Part model, mm, in its own coordinate system. A direction names the side the tool comes from. Coordinates: 2 decimals unless noted, no trailing zeros. Use a Markdown table: item, result. Add a question column.
1. 3-axis set-ups, long thin cutter, end or side, ignore diameter. For faces 1 (the flat face through (-29.4, 29.4, 43)), 2 (the flat face through (30.54, -12.3, -39.58)), 3 (the flat face through (37, 9, 0)): which of +Z, -Z, +X, -X, +Y, -Y reach the whole face in a straight line?
2. Drop flat-ended pins along their axis: pin 1 (6 mm diameter, centred on y = -10.5, z = -55, fed in from +X); pin 2 (8 mm diameter, centred on y = -9, z = -21, fed in from +X); pin 3 (1 mm diameter, centred on x = 2.5, y = -11.5, fed in from +Z). Give the stop position or say it passes through.
3. Pull direction Y, two halves, no side cores. Call faces 4 (the conical face through (-33.873, -25.973, 21.801)), 5 (the flat face through (-6.81, -32.21, -39.58)), 6 (the flat face through (0, -1, -83)): pulls with the +Y half, pulls with the -Y half, needs draft (parallel to the pull), parting line crosses it, or undercut.
4. Wall check: probe 1 along Y at (x, z) = (3.5, -10.5); probe 2 along Z at (x, y) = (-17, 12.5); probe 3 along X at (y, z) = (-12, -71). Give the ranges that are in metal, low to high. Write a range as [from, to].
from build123d import *

# Parameters (mm, degrees)
F1_DEPTH = 83
F1_TAPER = 3
F2_R     = 41.5426365129
F3_DEPTH = 43
F3_TAPER = -3
F4_T     = -2.5


with BuildPart() as f1:
    # F0 (on Top) → F1 (new body)
    with BuildSketch(Plane.XY):
        Polygon((29.8341157565, -26.5041046934), (39.8907686935, -1.126322166), (31.2820876222, 24.7784790206), (8.0361700908, 39.0891544913), (-18.9699607381, 35.109580148), (-37.0998361101, 14.7018430539), (-37.8702858474, -12.5850497979), (-20.9208079553, -33.983257982), (5.8177484879, -39.4803220745), align=None)
    extrude(amount=-F1_DEPTH, taper=F1_TAPER)

    # F2 (on Top) → F3 (join)
    with BuildSketch(Plane.XY):
        Circle(F2_R)
    extrude(amount=F3_DEPTH, taper=F3_TAPER)

    # F4
    f4_openings = [f1.faces().sort_by_distance(p)[0] for p in [
        (0, 0, 43),
    ]]
    offset(amount=F4_T, openings=f4_openings, kind=Kind.INTERSECTION)


solid = f1.part
Geometry check:
| question | item | result |
|---|---|---|
| 1 | face 1 | +Z, +X, -X, +Y, -Y |
| 1 | face 2 | +Z |
| 1 | face 3 | -Z |
| 2 | pin 1 | stops at x = 34.28 |
| 2 | pin 2 | stops at x = 37.19 |
| 2 | pin 3 | stops at z = -80.5 |
| 3 | face 4 | parting line crosses it |
| 3 | face 5 | undercut |
| 3 | face 6 | needs draft |
| 4 | probe 1 | y = [-38.44, -35.89], [35.33, 37.86] |
| 4 | probe 2 | z = [-83, -80.5] |
| 4 | probe 3 | x = [-33.59, -30.39], [28.89, 31.58] |
